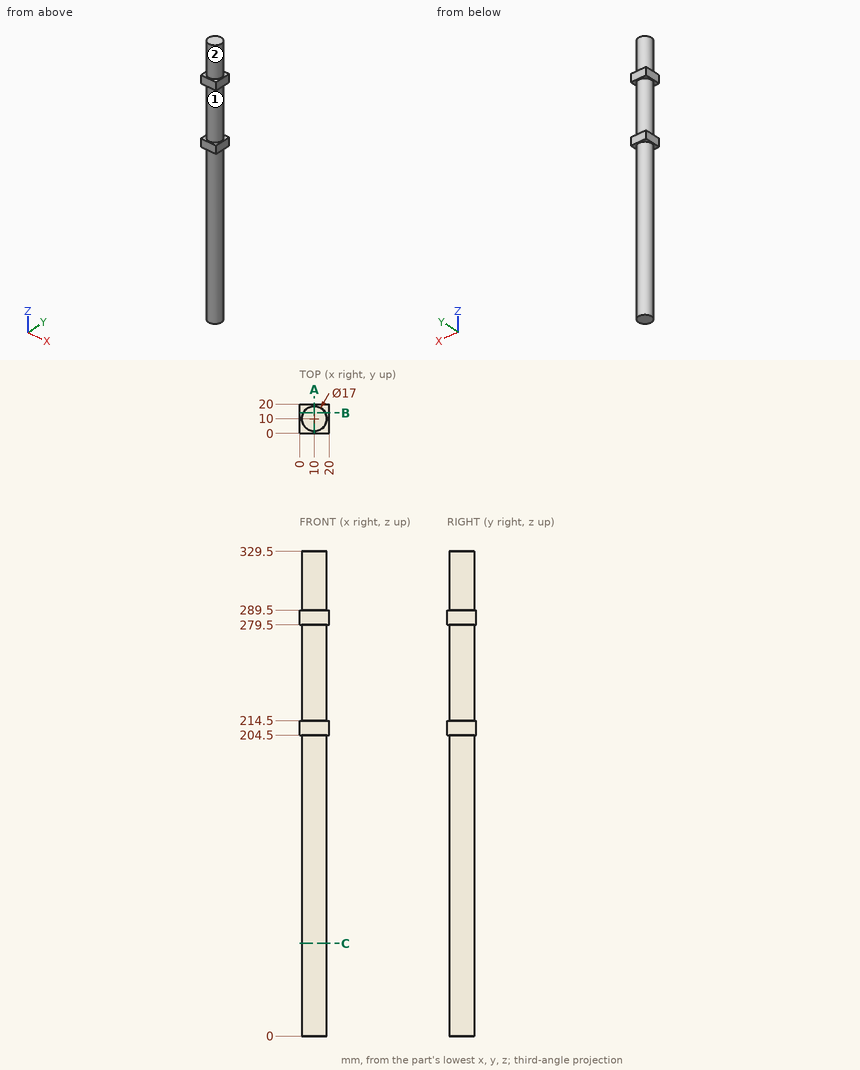
Geometry check sheet. Reference: drawing and pictorial views, mm from the part's lowest x, y, z. Round coordinates to 2 decimals unless told otherwise and drop trailing zeros. Order: outer loops, then holes, each group sorted by start corner. A loop starts at its lowest first (then second) coordinate and runs counter-clockwise, first axis right, second up. Notation, with made-up numbers: (68.25, 65.25) - (116.25, 65.25) arc R17 ccw to (116.25, 85.25) - close; hole circle Ø8 at (87.25, 88). An arc over 180 degrees is marked (long way). Use a Markdown table: item, result. Add a question column.
1) Section check B-B (y = 14). Record the cut outline in (x, z).
2) Gauge pin test, flat ends, axial feed: P1, Ø8, axis at x = 9.5, z = 84, coming from the -Y side; P2, Ø8, axis at x = 8.5, y = 6.5, coming from the -Z side; P3, Ø6, axis at y = 3.5, z = 99.5, coming from the +X side; P4, Ø2, axis at x = 6, z = 95.5, coming from the +Y side. Record the tip position at first contact, or that the pin passes through.
3) Thickness scan on line 1 along X through (y, z) = (10, 232); line 2 along Z through (x, y) = (3, 16.5); line 3 along Y through (x, z) = (10.75, 174.5). Record the ranges inside material, lowest first.
4) Section check A-A (x = 10). Record the cut outline in (y, z).
5) Section check C-C (z = 63). Record the cut outline in (x, y).
6) Mould release check, pull along Z, two halves, no side actions. Record for the marked faces 1 and 2: released by +Z, released by -Z, zero draft, split by the parting line, or undercut.
Established:
| question | item | result |
|---|---|---|
| 1 | outline | (0, 204.5) - (2.5, 204.5) - (2.5, 0) - (17.5, 0) - (17.5, 204.5) - (20, 204.5) - (20, 214.5) - (17.5, 214.5) - (17.5, 279.5) - (20, 279.5) - (20, 289.5) - (17.5, 289.5) - (17.5, 329.5) - (2.5, 329.5) - (2.5, 289.5) - (0, 289.5) - (0, 279.5) - (2.5, 279.5) - (2.5, 214.5) - (0, 214.5) - close |
| 2 | P1 | y = 1.5 |
| 2 | P2 | z = 0 |
| 2 | P3 | x = 17.75 |
| 2 | P4 | y = 17.95 |
| 3 | line 1 | 1.5 to 18.5 |
| 3 | line 2 | 204.5 to 214.5, 279.5 to 289.5 |
| 3 | line 3 | 1.53 to 18.47 |
| 4 | outline | (0, 204.5) - (1.5, 204.5) - (1.5, 0) - (18.5, 0) - (18.5, 204.5) - (20, 204.5) - (20, 214.5) - (18.5, 214.5) - (18.5, 279.5) - (20, 279.5) - (20, 289.5) - (18.5, 289.5) - (18.5, 329.5) - (1.5, 329.5) - (1.5, 289.5) - (0, 289.5) - (0, 279.5) - (1.5, 279.5) - (1.5, 214.5) - (0, 214.5) - close |
| 5 | outline | circle Ø17 at (10, 10) |
| 6 | face 1 | undercut |
| 6 | face 2 | zero draft |
